from build123d import *

# Parameters (mm, degrees)
ESQUISSE1_R        = 2.2
BOSS_EXTRU_1_DEPTH = 1.85
ESQUISSE2_R        = 1.25
BOSS_EXTRU_2_DEPTH = 3.8
CHANFREIN1_SIZE    = 1.85
CHANFREIN1_SIZE_2  = 0.3
CONG_1_R           = 0.1


with BuildPart() as part:
    # Esquisse1 → Boss.-Extru.1 (new body)
    with BuildSketch(Plane(origin=(0, 0, 0), x_dir=(1, 0, 0), z_dir=(0, 1, 0))):
        with Locations(Location((0, 0, 0), (0, 0, 270))):
            Circle(ESQUISSE1_R)
    extrude(amount=BOSS_EXTRU_1_DEPTH)

    # Esquisse2 → Boss.-Extru.2 (add)
    with BuildSketch(Plane(origin=(0, 1.85, 0), x_dir=(1, 0, 0), z_dir=(0, 1, 0))):
        with Locations(Location((0, 0, 0), (0, 0, 90))):
            Circle(ESQUISSE2_R)
    extrude(amount=BOSS_EXTRU_2_DEPTH)

    # Chanfrein1
    # the kernel refuses this chamfer: 1.85, 0.3 mm, written as the material it takes off along each edge
    with BuildSketch(Plane(origin=(0, 0, 0), x_dir=(0, 0, 1), z_dir=(-1, 0, 0))) as chanfrein1_piece_1:
        Polygon((2.2, CHANFREIN1_SIZE), (2.2 - CHANFREIN1_SIZE_2, 0), (2.2, 0), align=None)
    revolve(axis=Axis((0, 0, 0), (0, 1, 0)), mode=Mode.SUBTRACT)

    # Congé1
    cong_1_edges = [part.edges().sort_by_distance(p)[0] for p in [
        (0, 0, -1.9),
    ]]
    fillet(cong_1_edges, radius=CONG_1_R)


solid = part.part
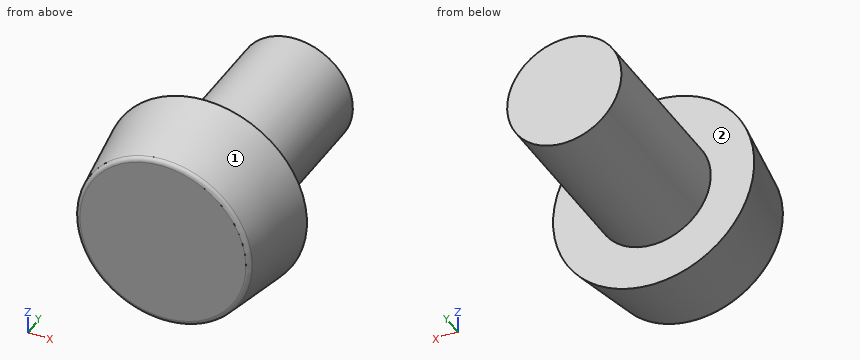
Here's how the part is built. I have some questions about the finished solid (model axes, mm). Face numbers are marked on the shaded views. A direction names the side the tool comes from. Round coordinates to 2 decimals unless told otherwise and drop trailing zeros. Write each loop counter-clockwise with the first axis right and the second up, starting at its lowest first coordinate (ties: lowest second). Pieces come first, ordered by that corner, then holes.
1. For the marked faces 1 and 2, which set-ups out of +Z, -Z, +X, -X, +Y, -Y let a thin tool reach every point of the face, with its end or its side?
2. Suppose I cut it at D-D (y = 1.65). List the corners of the cut face in (x, z) for me, and give its area (3 significant figures).
3. Suppose I cut it at A-A (z = 0). List the corners of the cut face in (x, y) for me, and give its area (3 significant figures).
4. Suppose I cut it at C-C (y = 3.4). List the corners of the cut face in (x, z) for me.
5. Suppose I cut it at B-B (x = 0). List the corners of the cut face in (y, z) for me, and give its area (3 significant figures).
6. I need wall thicknesses on L1, parallel to Y at x = -0.95, z = -1.45; L2, parallel to Z at x = 0.05, y = 5.25; L3, parallel to X at y = 4.35, z = -0.6. Which ranges of each line are inside material? Lowest first, please.
Answer sheet:
1. face 1: -Y
1. face 2: +Y
2. outline: circle Ø4.34 at (0, 0)
2. area: 14.8 mm2
3. outline: (-2.2, 1.85) - (-1.91, 0.08) arc R0.1 ccw to (-1.81, 0) - (1.81, 0) arc R0.1 ccw to (1.91, 0.08) - (2.2, 1.85) - (1.25, 1.85) - (1.25, 5.65) - (-1.25, 5.65) - (-1.25, 1.85) - close
3. area: 17.1 mm2
4. outline: circle Ø2.5 at (0, 0)
5. outline: (0, -1.81) arc R0.1 ccw to (0.08, -1.91) - (1.85, -2.2) - (1.85, -1.25) - (5.65, -1.25) - (5.65, 1.25) - (1.85, 1.25) - (1.85, 2.2) - (0.08, 1.91) arc R0.1 ccw to (0, 1.81) - close
5. area: 17.1 mm2
6. L1: y = 0 to 1.85
6. L2: z = -1.25 to 1.25
6. L3: x = -1.1 to 1.1
